Part model, mm, in its own coordinate system. Face numbers are marked on the shaded views. A direction names the side the tool comes from. Round coordinates to 2 decimals unless told otherwise and drop trailing zeros. Loops run counter-clockwise (first coordinate to the right, second up) from the corner with the lowest first, then second, coordinate; pieces in that order, holes last. Notation, with made-up numbers: (-19.75, -23) - (34.25, -23) arc R14 cw to (34.25, -12) - close; hole circle Ø9 at (39.25, 20.5). An arc over 180 degrees is marked (long way). Put each result on its own line as item: value.
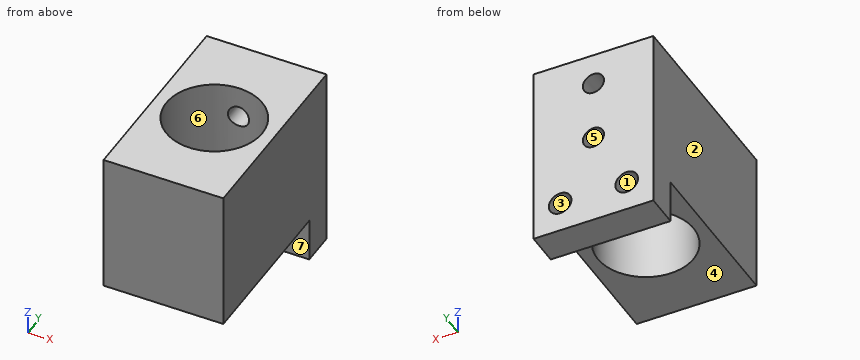
from build123d import *

# Parameters (mm, degrees)
SKETCH1_W                   = 22.86
SKETCH1_H                   = 35.56
BOSS_EXTRUDE1_DEPTH         = 38.1
SKETCH3_W                   = 22.86
SKETCH3_H                   = 8.382
CUT_EXTRUDE2_DEPTH          = 31.75
SKETCH4_R                   = 2.159
CUT_EXTRUDE3_DEPTH          = 6.35
SKETCH6_R                   = 9.144
CUT_EXTRUDE4_DEPTH          = 54.355116906
F_10_32_TAPPED_HOLE1_REACH  = 45.57
F_10_32_TAPPED_HOLE1_BORE_R = 2.0193


with BuildPart() as part:
    # Sketch1 → Boss-Extrude1 (new body)
    with BuildSketch(Plane(origin=(0, 0, 0), x_dir=(1, 0, 0), z_dir=(0, 1, 0))):
        Rectangle(SKETCH1_W, SKETCH1_H)
    extrude(amount=BOSS_EXTRUDE1_DEPTH)

    # Sketch3 → Cut-Extrude2 (cut)
    with BuildSketch(Plane.XZ):
        with Locations((0, -13.589)):
            Rectangle(SKETCH3_W, SKETCH3_H)
    extrude(amount=-CUT_EXTRUDE2_DEPTH, mode=Mode.SUBTRACT)

    # Sketch4 → Cut-Extrude3 (cut)
    with BuildSketch(Plane(origin=(0, 38.1, 0), x_dir=(1, 0, 0), z_dir=(0, 1, 0))):
        with Locations(Location((-6.35, 11.938, 0), (0, 0, 270))):
            Circle(SKETCH4_R)
        with Locations(Location((6.35, 11.938, 0), (0, 0, 90))):
            Circle(SKETCH4_R)
    extrude(amount=-CUT_EXTRUDE3_DEPTH, mode=Mode.SUBTRACT)

    # Sketch6 → Cut-Extrude4 (cut, through all)
    with BuildSketch(Plane.XY.offset(17.78)):
        with Locations((0, 18.796)):
            Circle(SKETCH6_R)
    extrude(amount=-CUT_EXTRUDE4_DEPTH, mode=Mode.SUBTRACT)

    # #10-32 Tapped Hole1 bore → #10-32 Tapped Hole1 (cut, up to next)
    with BuildSketch(Plane(origin=(0, 38.1, 0), x_dir=(1, 0, 0), z_dir=(0, 1, 0)), mode=Mode.PRIVATE) as f_10_32_tapped_hole1_sk1:
        Circle(F_10_32_TAPPED_HOLE1_BORE_R)
    f_10_32_tapped_hole1_tool1 = extrude(f_10_32_tapped_hole1_sk1.sketch, amount=-F_10_32_TAPPED_HOLE1_REACH, mode=Mode.PRIVATE) & part.part
    # #10-32 Tapped Hole1 bore → #10-32 Tapped Hole1 (cut, up to next)
    with BuildSketch(Plane(origin=(0, 38.1, 0), x_dir=(1, 0, 0), z_dir=(0, 1, 0)), mode=Mode.PRIVATE) as f_10_32_tapped_hole1_sk2:
        with Locations((0, -11.689474191)):
            Circle(F_10_32_TAPPED_HOLE1_BORE_R)
    f_10_32_tapped_hole1_tool2 = extrude(f_10_32_tapped_hole1_sk2.sketch, amount=-F_10_32_TAPPED_HOLE1_REACH, mode=Mode.PRIVATE) & part.part
    add(f_10_32_tapped_hole1_tool1.solids().sort_by_distance((0, 38.1, 0))[0], mode=Mode.SUBTRACT)
    add(f_10_32_tapped_hole1_tool2.solids().sort_by_distance((0, 38.1, 11.689474))[0], mode=Mode.SUBTRACT)


solid = part.part
1. Pin check, flat tips, straight feed: P1, Ø2, axis at x = 1.5, y = 26.5, coming from the +Z side; P2, Ø2.5, axis at x = 0, z = 0, coming from the +Y side; P3, Ø8, axis at x = -8.5, y = 11.5, coming from the -Z side; P4, Ø4, axis at x = -2.5, z = -14.5, coming from the -Y side. Stop position of each tip, or through.
A:
P1: passes through
P2: stops at y = 9.74
P3: stops at z = -9.4
P4: stops at y = 31.75
2. Band-saw the part on C-C (z = 0). List the corners of the cut face in (x, y), plus the area to 3 significant figures.
A:
outline: (-11.43, 0) - (11.43, 0) - (11.43, 38.1) - (2.02, 38.1) - (2.02, 27.71) arc R9.14 cw (long way) to (-2.02, 27.71) - (-2.02, 38.1) - (-11.43, 38.1) - close
area: 567 mm²
3. Probe line 1 along Z through (x, y) = (0, 33.75); line 2 along Z through (x, y) = (-4.5, 8); line 3 along Y through (x, z) = (6, 15.5). List the from-to ranges inside material, lowest first. Write a range as [from, to].
A:
line 1: z = [-17.78, -2.02], [2.02, 9.67], [13.71, 17.78]
line 2: z = [-9.4, 17.78]
line 3: y = [0, 11.9], [25.7, 38.1]
4. Band-saw the part on D-D (x = 3). List the corners of the cut face in (y, z), plus the area to 3 significant figures.
A:
outline: (0, -9.4) - (10.16, -9.4) - (10.16, 17.78) - (0, 17.78) - close; (27.43, -9.4) - (31.75, -9.4) - (31.75, -17.78) - (38.1, -17.78) - (38.1, 17.78) - (27.43, 17.78) - close
area: 619 mm²
5. Two-plate mould, pull along Z, no slides. Class the marked faces 1, 2, 3 and 4: pulls with the +Z half, pulls with the -Z half, needs draft (parallel to the pull), parting line crosses it, or undercut.
A:
face 1: undercut
face 2: needs draft
face 3: undercut
face 4: pulls with the -Z half
6. Band-saw the part on A-A (x = 0). List the corners of the cut face in (y, z), plus the area to 3 significant figures.
A:
outline: (0, -9.4) - (9.65, -9.4) - (9.65, 17.78) - (0, 17.78) - close; (27.94, -9.4) - (31.75, -9.4) - (31.75, -17.78) - (38.1, -17.78) - (38.1, -2.02) - (27.94, -2.02) - close; (27.94, 2.02) - (38.1, 2.02) - (38.1, 9.67) - (27.94, 9.67) - close; (27.94, 13.71) - (38.1, 13.71) - (38.1, 17.78) - (27.94, 17.78) - close
area: 510 mm²
7. Band-saw the part on B-B (y = 21.5). List the corners of the cut face in (x, z).
A:
outline: (-11.43, -9.4) - (-8.74, -9.4) - (-8.74, 17.78) - (-11.43, 17.78) - close; (8.74, -9.4) - (11.43, -9.4) - (11.43, 17.78) - (8.74, 17.78) - close
8. Tool access for the marked faces 5, 6 and 7: list every direction of +Z, -Z, +X, -X, +Y, -Y with a clear straight run to the whole face (end or side of a thin tool).
A:
face 5: +Y
face 6: +Z, -Z
face 7: -Z, +X, -X, -Y
